Design review of the part built by this model. Coordinates are the model's own, in mm. Give positions to 0.01 mm unless a question says otherwise; leave off trailing zeros. Loops run counter-clockwise (first coordinate to the right, second up) from the corner with the lowest first, then second, coordinate; pieces in that order, holes last. Notation, with made-up numbers: M 23,47 L 28,47 A20 ccw 28,57 Z; hole C 77.5,40 d9. An arc over 180 degrees is marked long. Use a Markdown table: item, result. Add a question column.
(1) Add section C-C, the plane x = -10.5. Give the boundary of the cut face in (y, z), then the cut area to 3 significant figures.
(2) Insertion check: pin 1 Ø1.5 at (x, z) = (20, -8.5) entering from -Y; pin 2 Ø3 at (x, z) = (28.97, -40.94) entering from -Y. Each pin has a flat end and moves straight along its axis. Give the tip position at first contact, or say it passes through.
(3) Add section B-B, the plane y = 1.75. State how many separate pieces and enclosed holes the cut face has, then the cut area to 3 significant figures.
(4) Add section A-A, the plane x = 0. Give the boundary of the cut face in (y, z).
(5) For probe 1 along X at (y, z) = (2.25, -41.5); probe 2 along X at (y, z) = (1, -53.5); probe 3 along Z at (x, y) = (28, 2.95), list the stretches that pass through material, from the lowest coordinate up.
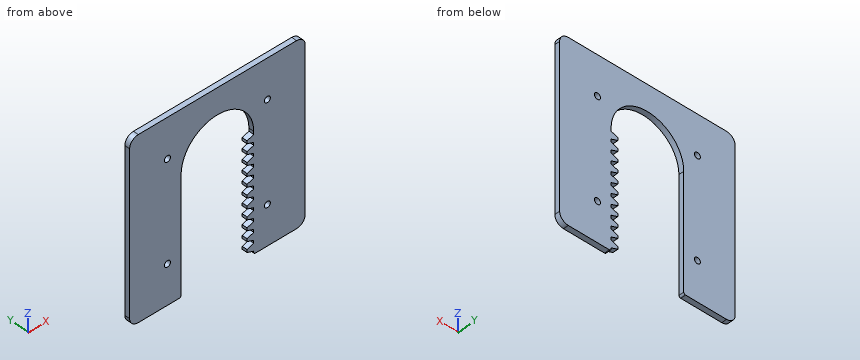
```python
from build123d import *

# Parameters (mm, degrees)
SKETCH1_R           = 1.75
BOSS_EXTRUDE1_DEPTH = 3


with BuildPart() as part:
    # Sketch1 → Boss-Extrude1 (new body)
    with BuildSketch(Plane(origin=(0, 0, 0), x_dir=(1, 0, 0), z_dir=(0, 1, 0))):
        with BuildLine():
            Line((21.058452488, 3.842990858), (17.188733854, 5.16651258))
            Line((17.188733854, 5.16651258), (17.188733854, 6.83348742))
            Line((17.188733854, 6.83348742), (21.058452488, 8.157009142))
            Line((21.058452488, 8.157009142), (21.058452488, 9.842990858))
            Line((21.058452488, 9.842990858), (17.188733854, 11.16651258))
            Line((17.188733854, 11.16651258), (17.188733854, 12.83348742))
            Line((17.188733854, 12.83348742), (21.058452488, 14.157009142))
            Line((21.058452488, 14.157009142), (21.058452488, 15.842990858))
            Line((21.058452488, 15.842990858), (17.188733854, 17.16651258))
            Line((17.188733854, 17.16651258), (17.188733854, 18.83348742))
            Line((17.188733854, 18.83348742), (21.058452488, 20.157009142))
            Line((21.058452488, 20.157009142), (21.058452488, 21.842990858))
            Line((21.058452488, 21.842990858), (17.188733854, 23.16651258))
            Line((17.188733854, 23.16651258), (17.188733854, 24.83348742))
            Line((17.188733854, 24.83348742), (21.058452488, 26.157009142))
            Line((21.058452488, 26.157009142), (21.058452488, 27.842990858))
            Line((21.058452488, 27.842990858), (17.188733854, 29.16651258))
            Line((17.188733854, 29.16651258), (17.188733854, 30.83348742))
            Line((17.188733854, 30.83348742), (21.058452488, 32.157009142))
            Line((21.058452488, 32.157009142), (21.058452488, 33.842990858))
            Line((21.058452488, 33.842990858), (17.188733854, 35.16651258))
            Line((17.188733854, 35.16651258), (17.188733854, 36.83348742))
            Line((17.188733854, 36.83348742), (21.058452488, 38.157009142))
            Line((21.058452488, 38.157009142), (21.058452488, 39.842990858))
            Line((21.058452488, 39.842990858), (17.188733854, 41.16651258))
            Line((17.188733854, 41.16651258), (17.188733854, 42.83348742))
            Line((17.188733854, 42.83348742), (21.058452488, 44.157009142))
            Line((21.058452488, 44.157009142), (21.058452488, 45.842990858))
            Line((21.058452488, 45.842990858), (17.188733854, 47.16651258))
            Line((17.188733854, 47.16651258), (17.188733854, 48.83348742))
            Line((17.188733854, 48.83348742), (21.058452488, 50.157009142))
            Line((21.058452488, 50.157009142), (21.058452488, 51.842990858))
            Line((21.058452488, 51.842990858), (17.188733854, 53.16651258))
            Line((17.188733854, 53.16651258), (17.188733854, 54.83348742))
            Line((17.188733854, 54.83348742), (21.058452488, 56.157009142))
            Line((21.058452488, 56.157009142), (21.058452488, 57.842990858))
            Line((21.058452488, 57.842990858), (17.188733854, 59.16651258))
            Line((17.188733854, 59.16651258), (17.188733854, 60.83348742))
            Line((17.188733854, 60.83348742), (21.058452488, 62.157009142))
            Line((21.058452488, 62.157009142), (21.058452488, 62.842990858))
            ThreePointArc((21.058452488, 62.842990858), (21.351345707, 63.550097639), (22.058452488, 63.842990858))
            Line((22.058452488, 63.842990858), (45.872217102, 63.842990858))
            ThreePointArc((45.872217102, 63.842990858), (49.407751008, 62.378524764), (50.872217102, 58.842990858))
            Line((50.872217102, 58.842990858), (50.872217102, -34.901443346))
            ThreePointArc((50.872217102, -34.901443346), (49.407751008, -38.436977252), (45.872217102, -39.901443346))
            Line((45.872217102, -39.901443346), (-45.872217102, -39.901443346))
            ThreePointArc((-45.872217102, -39.901443346), (-49.407751008, -38.436977252), (-50.872217102, -34.901443346))
            Line((-50.872217102, -34.901443346), (-50.872217102, 58.842990858))
            ThreePointArc((-50.872217102, 58.842990858), (-49.407751008, 62.378524764), (-45.872217102, 63.842990858))
            Line((-45.872217102, 63.842990858), (-22.058452488, 63.842990858))
            ThreePointArc((-22.058452488, 63.842990858), (-21.351345707, 63.550097639), (-21.058452488, 62.842990858))
            Line((-21.058452488, 62.842990858), (-21.058452488, -3.842990858))
            ThreePointArc((-21.058452488, -3.842990858), (0, -24.901443346), (21.058452488, -3.842990858))
            Line((21.058452488, -3.842990858), (21.058452488, -2.157009142))
            Line((21.058452488, -2.157009142), (17.188733854, -0.83348742))
            Line((17.188733854, -0.83348742), (17.188733854, 0.83348742))
            Line((17.188733854, 0.83348742), (21.058452488, 2.157009142))
            Line((21.058452488, 2.157009142), (21.058452488, 3.842990858))
        make_face()
        with Locations(Location((28.965334795, -16.994561039, 0), (0, 0, 270))):
            Circle(SKETCH1_R, mode=Mode.SUBTRACT)
        with Locations(Location((-28.965334795, -16.994561039, 0), (0, 0, 270))):
            Circle(SKETCH1_R, mode=Mode.SUBTRACT)
        with Locations(Location((-28.965334795, 40.936108551, 0), (0, 0, 270))):
            Circle(SKETCH1_R, mode=Mode.SUBTRACT)
        with Locations(Location((28.965334795, 40.936108551, 0), (0, 0, 270))):
            Circle(SKETCH1_R, mode=Mode.SUBTRACT)
    extrude(amount=BOSS_EXTRUDE1_DEPTH)


solid = part.part
```
Established:
| question | item | result |
|---|---|---|
| 1 | outline | M 0,22.1 L 3,22.1 L 3,39.9 L 0,39.9 Z |
| 1 | area | 53.4 mm^2 |
| 2 | pin 1 | y = 0 |
| 2 | pin 2 | through |
| 3 | separate pieces | 1 |
| 3 | enclosed holes | 4 |
| 3 | area | 7,080 mm^2 |
| 4 | outline | M 0,24.9 L 3,24.9 L 3,39.9 L 0,39.9 Z |
| 5 | probe 1 | -50.87 to -30.62, -27.31 to -21.06, 17.19 to 27.31, 30.62 to 50.87 |
| 5 | probe 2 | -50.87 to -21.06, 17.19 to 50.87 |
| 5 | probe 3 | -63.84 to -42.4, -39.48 to 15.53, 18.45 to 39.9 |
